from build123d import *

# Parameters (mm, degrees)
F0_R     = 7.9375
F0_R_2   = 6.35
F0_R_3   = 4.7625
F1_DEPTH = 3
F2_DEPTH = 15.875
F3_R     = 0.508


with BuildPart() as f1:
    # F0 (on Top) → F1 (new body)
    with BuildSketch(Plane.XY):
        Circle(F0_R)
        Circle(F0_R_2, mode=Mode.SUBTRACT)
        Circle(F0_R_2)
        Circle(F0_R_3, mode=Mode.SUBTRACT)
    extrude(amount=-F1_DEPTH)

    # F0 (on Top) → F2 (join)
    with BuildSketch(Plane.XY):
        Circle(F0_R_2)
        Circle(F0_R_3, mode=Mode.SUBTRACT)
    extrude(amount=F2_DEPTH)

    # F3
    f3_edges = [f1.edges().sort_by_distance(p)[0] for p in [
        (-4.7625, 0, 15.875),
    ]]
    fillet(f3_edges, radius=F3_R)


solid = f1.part
Could you check a few things on this model? Use its own coordinates, in mm. A direction names the side the tool comes from. Give positions to 0.01 mm unless a question says otherwise; leave off trailing zeros. Loops run counter-clockwise (first coordinate to the right, second up) from the corner with the lowest first, then second, coordinate; pieces in that order, holes last. Notation, with made-up numbers: (21.5, -6) -> (72.5, -6) arc R30 ccw to (72.5, 16) -> close; hole circle Ø1 at (19, 65.5). An arc over 180 degrees is marked (long way). Return JSON: item names as keys, results as strings.
Item 1: If we section it at D-D on y = 6: List the corners of the cut face in (x, z) for me (3 decimals).
Geometry results:
{"outline": "(-5.197, -3) -> (5.197, -3) -> (5.197, 0) -> (2.079, 0) -> (2.079, 15.875) -> (-2.079, 15.875) -> (-2.079, 0) -> (-5.197, 0) -> close"}
Item 2: If we section it at C-C on z = -0.5: List the corners of the cut face in (x, y) for me (1 decimal), plus the area to 3 significant figures.
Geometry results:
{"outline": "circle Ø15.9 at (0, 0); hole circle Ø9.5 at (0, 0)", "area": "127 mm²"}
Item 3: I'm going to push flat-ended pins straight in: pin 1 (8 mm diameter, centred on y = -5.5, z = 10.5, fed in from -X); pin 2 (3 mm diameter, centred on x = -5, z = 5, fed in from +Y); pin 3 (7.5 mm diameter, centred on x = 0, y = 0, fed in from +Z); pin 4 (2 mm diameter, centred on y = -5.5, z = 0.5, fed in from +X). Where does each tip first touch, or does it pass through?
Geometry results:
{"pin 1": "stops at x = -6.17", "pin 2": "stops at y = 5.3", "pin 3": "passes through", "pin 4": "stops at x = 6.44"}
Item 4: Which directions (+Z, -Z, +X, -X, +Y, -Y) give clear straight access to the entire face, cutting with the end or side of a thin tool? Please do faces 1 (the cylindrical face through (-1.38, -6.2, 7.83)), 2 (the flat face through (-4, 4, 15.875)).
Geometry results:
{"face 1": "+Z", "face 2": "+Z, +X, -X, +Y, -Y"}
Item 5: I need wall thicknesses on L1, parallel to Y at x = 0, z = 7.75; L2, parallel to Z at x = -5, y = -4.75; L3, parallel to Y at x = -1.25, z = 4. Which ranges of each line are inside material? Lowest first, please. Write a range as from..to.
Geometry results:
{"L1": "y = -6.35..-4.76, 4.76..6.35", "L2": "z = -3..0", "L3": "y = -6.23..-4.6, 4.6..6.23"}
